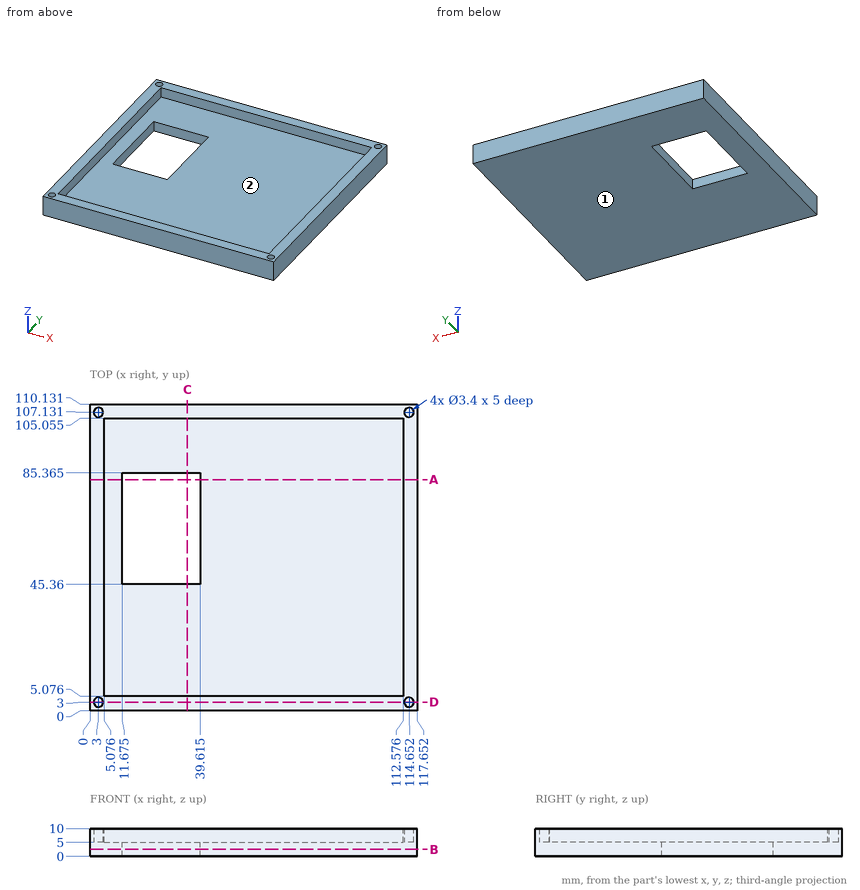
Geometry: see drawing. Coordinates: mm, zero at the bounding-box minimum. Round coordinates to 2 decimals unless told otherwise and drop trailing zeros. Write each loop counter-clockwise with the first axis right and the second up, starting at its lowest first coordinate (ties: lowest second). Pieces come first, ordered by that corner, then holes. Notation, with made-up numbers: M 56.5,-27.5 L 110.5,-27.5 A13 ccw 110.5,-21.5 Z; hole C 47.25,-3 d9. An arc over 180 degrees is marked long. Answer in a Markdown table with one row per item. Add a question column.
(1) Cut plane C-C, the plane x = 35. Return the cut outline in (y, z) (1 decimal).
(2) Cut plane A-A, the plane y = 83. Return the cut outline in (x, z) (1 decimal), then the cut area to 3 significant figures.
(3) Contact query for a flat-ended pin moving along its axis: pin 1 (2.5 mm diameter, centred on x = 115, y = 3, fed in from +Z). Output: stop coordinate, or through.
(4) Draft query along X for the marked faces 1 and 2. Return one class per face: pulls with the +X half, pulls with the -X half, needs draft (parallel to the pull), parting line crosses it, or undercut.
(5) Ray query, L1, parallel to Y at x = 3, z = 8.5; L2, parallel to Y at x = 104, z = 8.25 (1 decimal); L3, parallel to X at y = 81, z = 8. Return the intervals inside material, ascending.
(6) Cut plane D-D, the plane y = 3. Return the cut outline in (x, z), then the cut area to 3 significant figures.
(7) Cut plane B-B, the plane z = 2.5. Return the cut outline in (x, y) (1 decimal).
Established:
| question | item | result |
|---|---|---|
| 1 | outline | M 0,0 L 45.4,0 L 45.4,5 L 5.1,5 L 5.1,10 L 0,10 Z; M 85.4,0 L 110.1,0 L 110.1,10 L 105.1,10 L 105.1,5 L 85.4,5 Z |
| 2 | outline | M 0,0 L 11.7,0 L 11.7,5 L 5.1,5 L 5.1,10 L 0,10 Z; M 39.6,0 L 117.7,0 L 117.7,10 L 112.6,10 L 112.6,5 L 39.6,5 Z |
| 2 | area | 499 mm² |
| 3 | pin 1 | z = 5 |
| 4 | face 1 | needs draft |
| 4 | face 2 | undercut |
| 5 | L1 | 0 to 1.3, 4.7 to 105.43, 108.83 to 110.13 |
| 5 | L2 | 0 to 5.1, 105.1 to 110.1 |
| 5 | L3 | 0 to 5.08, 112.58 to 117.65 |
| 6 | outline | M 0,0 L 117.65,0 L 117.65,10 L 116.35,10 L 116.35,5 L 112.95,5 L 112.95,10 L 4.7,10 L 4.7,5 L 1.3,5 L 1.3,10 L 0,10 Z |
| 6 | area | 1,140 mm² |
| 7 | outline | M 0,0 L 117.7,0 L 117.7,110.1 L 0,110.1 Z; hole M 11.7,45.4 L 39.6,45.4 L 39.6,85.4 L 11.7,85.4 Z |
